Input: part model. Units: mm. Frame: model coordinates. Face numbers are marked on the shaded views. A direction names the side the tool comes from. Coordinates: 2 decimals unless noted, no trailing zeros. Use CSV: the item, a comma, the result in double quotes. Start each with the question number.
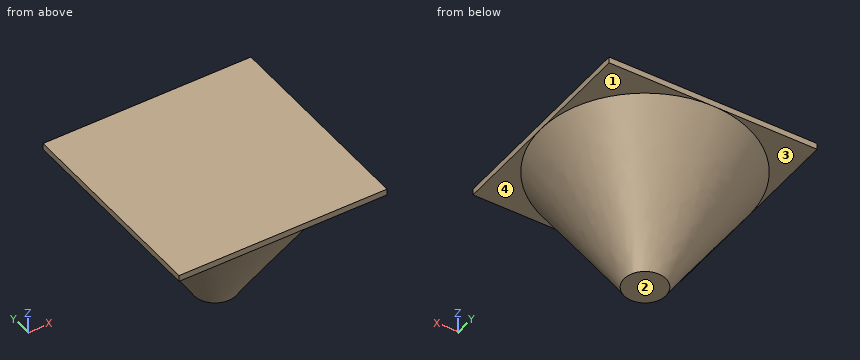
```python
from build123d import *

# Parameters (mm, degrees)
EXTRUDE_1_DEPTH = 15


with BuildPart() as part:
    # 放样1: read off the stored shape, not the designer's step
    # 放样1: loft between two sections, ruled curve by curve
    loft_1_from = [
        Edge.make_bspline([(157.289403045, 194.319437241, 300), (545.928277528, -120.259368848, 300), (231.349471438, -508.898243331, 300), (-157.289403045, -194.319437241, 300), (-545.928277528, 120.259368848, 300), (-231.349471438, 508.898243331, 300), (157.289403045, 194.319437241, 300)], [0, 0, 0, 0, 0.5, 0.5, 0.5, 1, 1, 1, 1], 3, [1, 0.333333333, 0.333333333, 1, 0.333333333, 0.333333333, 1]),
    ]
    loft_1_to = [
        Edge.make_bspline([(42.317097013, 26.631997679, 0), (95.581092372, -58.002196347, 0), (10.946898346, -111.266191705, 0), (-42.317097013, -26.631997679, 0), (-95.581092372, 58.002196347, 0), (-10.946898346, 111.266191705, 0), (42.317097013, 26.631997679, 0)], [0, 0, 0, 0, 0.5, 0.5, 0.5, 1, 1, 1, 1], 3, [1, 0.333333333, 0.333333333, 1, 0.333333333, 0.333333333, 1]),
    ]
    loft_1 = Solid(Shell([*[Face.make_surface_from_curves(loft_1_from[k], loft_1_to[k]) for k in range(1)], Face(Wire(loft_1_from)), Face(Wire(loft_1_to))]))
    add(loft_1)

    # 草图4 → 凸台-拉伸1 (add)
    with BuildSketch(Plane.XY.offset(300)):
        Polygon((0, 250), (-250, 250), (-250, -250), (250, -250), (250, 250), align=None)
    extrude(amount=EXTRUDE_1_DEPTH)


solid = part.part
```
1. Access query for the marked faces 1, 2, 3 and 4. Directions: +Z, -Z, +X, -X, +Y, -Y. A direction counts if a zero-diameter tool reaches every point of the face in a straight line with its end or side. Return the directions, or none.
2. Contact query for flat-ended pins moving along their axis: P1, Ø1, axis at x = -26.5, y = -129.5, coming from the -Z side; P2, Ø5, axis at y = 61, z = 197, coming from the -X side; P3, Ø4, axis at x = 136, z = 178.5, coming from the +Y side. Output: stop coordinate, or through.
3. Material intervals for line 1 along Z through (x, y) = (221, -205.5); line 2 along Z through (x, y) = (-10, 68); line 3 along X through (y, z) = (166, 252), sorted ascending.
Values follow:
1,face 1,"-Z, +X, +Y"
1,face 2,"-Z, +X, -X, +Y, -Y"
1,face 3,"-Z, -X, +Y"
1,face 4,"-Z, +X, -Y"
2,P1,"stops at z = 124.37"
2,P2,"stops at x = -171.87"
2,P3,"stops at y = 102.22"
3,line 1,"z = 300 to 315"
3,line 2,"z = 29.38 to 315"
3,line 3,"x = -140.67 to 140.67"
